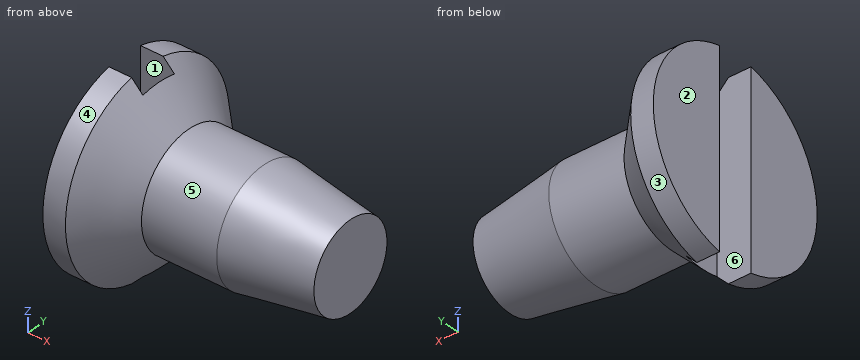
Autodesk Inventor part; units mm, degrees
ref_plane "Work Plane1" through (2.2553, 0, 0) normal (0, 0, -1) x (1, 0, 0)
ref_plane "YZ Plane" through (0, 0, 0) normal (1, 0, 0) x (0, 1, 0)
ref_plane "XZ Plane" through (0, 0, 0) normal (0, 1, 0) x (-1, 0, 0)
sketch "Sketch1" plane through (0, 0, 0) normal (0, 0, 1) x (1, 0, 0)
  line L0 (-1.2, 0) -> (7.2, 0)
  line L1 (0, 0) -> (6, 0)
  line L2 (6, 0) -> (6, 1.5)
  line L3 (6, 1.5) -> (1.7, 1.5)
  line L4 (1.7, 1.5) -> (1.7, 1.5)
  line L5 (1.7, 1.5) -> (0.6, 2.6)
  line L6 (0.6, 2.6) -> (0, 2.6)
  line L7 (0, 2.6) -> (0, 0)
  line L8 (0, -0.52) -> (0, 3.12)
  dimension "d0" = 6
  dimension "d1" = 1.7
  dimension "d2" = 3
  dimension "d3" = 3
  dimension "d4" = 5.2
  dimension "d5" = 45
revolve "Body" add sketch "Sketch1" angle 360 about axis through (0, 0, 0) along (1, 0, 0)
sketch "Sketch2" plane through (0, 0, 0) normal (-1, 0, 0) x (0, 0, 1)
  circle A0 centre (0, 0) radius 2.6
  line L0 (-3.64, 0) -> (3.64, 0)
  line L1 (-2.6, 0) -> (-2.6, 0.5)
  line L2 (-2.6, 0.5) -> (2.6, 0.5)
  line L3 (2.6, 0) -> (2.6, 0.5)
  line L4 (-2.6, 0) -> (-2.6, -0.5)
  line L5 (-2.6, -0.5) -> (2.6, -0.5)
  line L6 (2.6, 0) -> (2.6, -0.5)
  dimension "d8" = 1
extrude "Slot" cut sketch "Sketch2" against normal blind 0.9 contours L0 A0 L2 | L6 L5 A0 | A0 L5 L0 | A0 L2 L3 | L1 L2 A0 | A0 L5 L4
thread "Thread"
chamfer "Chamfer1" distance 0.34 distance2 2.3 1 edges at (6, -1.5, 0) measured on face at (6, -0.8773, -0.3972)
ref_plane "Work Plane1" through (2.2553, 0, 0) normal (0, 0, -1) x (1, 0, 0)
equation "\"d8\" = SBR"
equation "\"d9\" = STI"
equation "\"d0\" = NLG"
equation "\"d1\" = KOH"
equation "\"d2\" = NND"
equation "\"d3\" = SED2"
equation "\"d4\" = KOD"
equation "\"d5\" = 0.5 * SEWI"
equation "\"d6\" = GEL"
equation "\"d14\" = -0.5 * GD2 + 0.5 * NND"
equation "\"d15\" = SPTZ"
equation "\"NND\" = 3"
equation "\"NLG\" = 6"
equation "\"GEL\" = 4.3"
equation "\"KOH\" = 1.7"
equation "\"KOD\" = 5.2"
equation "\"SBR\" = 1"
equation "\"STI\" = 0.9"
equation "\"GD2\" = 2.32"
equation "\"SED2\" = 3"
equation "\"SEWI\" = 90deg"
equation "\"SPTZ\" = 2.3"
equation "\"GUL\" = 0.61345 * PTC"
equation "\"THREADDIA\" = 3"
equation "\"TOA\" = 30deg"
equation "\"PTC\" = 0.5"
equation "\"GAL\" = 0.61345 * PTC"
equation "\"GD1\" = THREADDIA - 1.2269 * PTC"
properties part number "ANSI/ASME B18.6.5M - M3x0.5 x 6, SFCHTSTTM" material "Steel, Mild"
Build history of the part. All positions in model axes, mm. Face numbers are marked on the shaded views. A direction names the side the tool comes from. Coordinates: 2 decimals unless noted, no trailing zeros. Order: outer loops, then holes, each group sorted by start corner. A loop starts at its lowest first (then second) coordinate and runs counter-clockwise, first axis right, second up. Notation, with made-up numbers: (89, 9) - (106, 9) arc R22 ccw to (106, 25) - close; hole circle Ø2 at (17, 71.25). An arc over 180 degrees is marked (long way). Write item = value, one per line. Start each with the question number.
1) Saw through at D-D on x = 1.5. Write the cut outline in (y, z), then the cut area to 3 significant figures.
2) Flat gauge pins, fed straight in: pin 1 Ø1 at (x, z) = (0.5, 1) entering from +Y; pin 2 Ø3 at (y, z) = (0.5, -0.5) entering from -X; pin 3 Ø1 at (x, y) = (1.5, 1) entering from -Z; pin 4 Ø1.5 at (x, y) = (5, -1) entering from +Z. Where does each tip first touch, or does it go through?
3) 3-axis set-ups, long thin cutter, end or side, ignore diameter. For the marked faces 4, 5 and 6: which of +Z, -Z, +X, -X, +Y, -Y reach the whole face in a straight line?
4) Wall check: line 1 along X through (y, z) = (0.05, 0.05); line 2 along Y through (x, z) = (2.25, -0.8); line 3 along Z through (x, y) = (5.75, 0.3). Give the ranges that are in metal, low to high. Write a range as from..to.
5) Saw through at A-A on y = 0. Write the cut outline in (x, z).
6) Two-plate mould, pull along Y, no slides. Class the marked faces 1, 2 and 3: pulls with the +Y half, pulls with the -Y half, needs draft (parallel to the pull), parting line crosses it, or undercut.
7) Saw through at C-C on x = 0.75. Write the cut outline in (y, z).
8) Saw through at B-B on z = 0. Write the cut outline in (x, y).
From the geometry:
q1.outline = circle Ø3.4 at (0, 0)
q1.area = 9.08 mm^2
q2.pin_1 = 2.55
q2.pin_2 = 0
q2.pin_3 = -2.01
q2.pin_4 = 1.32
q3.face_4 = +X, -X, -Y
q3.face_5 = +X
q3.face_6 = +Z, -Z, -X
q4.line_1 = 0.9..6
q4.line_2 = -1.27..1.27
q4.line_3 = -1.16..1.16
q5.outline = (0.9, -2.3) - (1.7, -1.5) - (3.7, -1.5) - (6, -1.16) - (6, 1.16) - (3.7, 1.5) - (1.7, 1.5) - (0.9, 2.3) - close
q6.face_1 = undercut
q6.face_2 = needs draft
q6.face_3 = pulls with the +Y half
q7.outline = (-0.5, -2.4) - (-0.5, 2.4) arc R2.45 ccw to start; (0.5, -2.4) arc R2.45 ccw to (0.5, 2.4) - close
q8.outline = (0, -2.6) - (0.6, -2.6) - (1.7, -1.5) - (3.7, -1.5) - (6, -1.16) - (6, 1.16) - (3.7, 1.5) - (1.7, 1.5) - (0.6, 2.6) - (0, 2.6) - (0, 0.5) - (0.9, 0.5) - (0.9, -0.5) - (0, -0.5) - close
